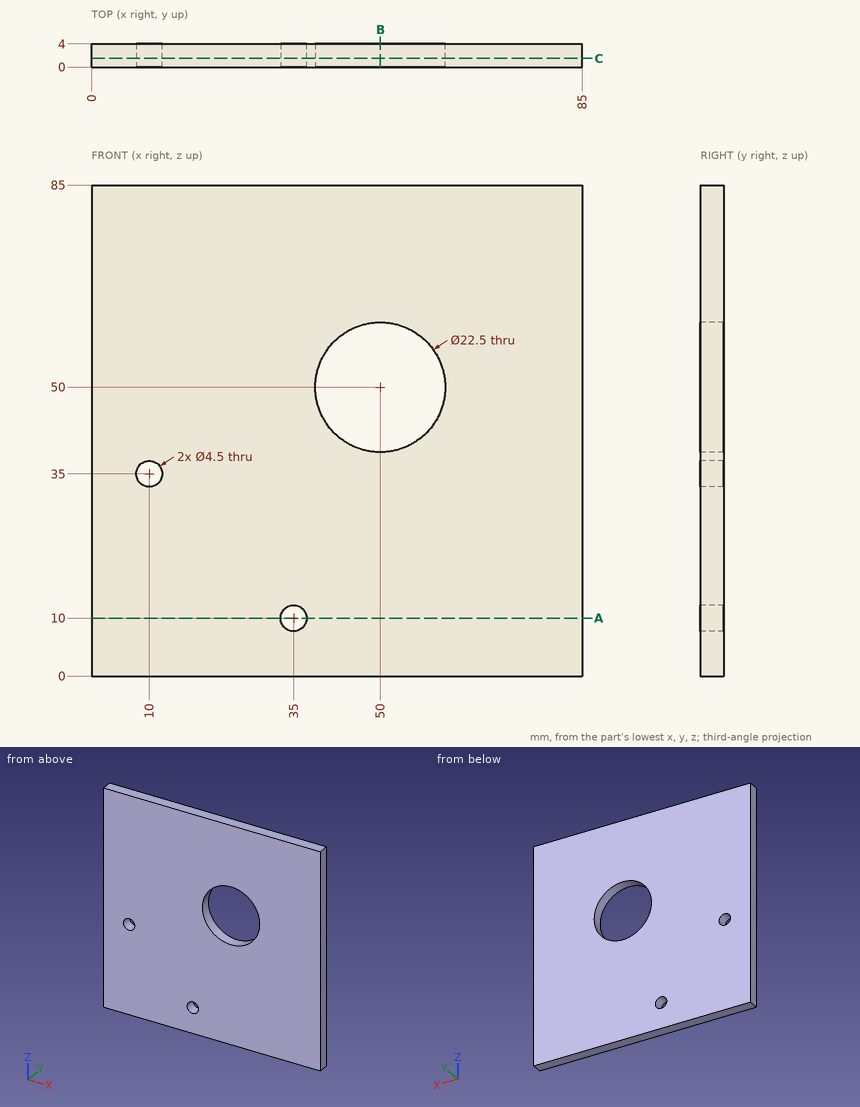
Here's the drawing with two shaded views (mm, measured from the low corner). I have some questions. Coordinates: 2 decimals unless noted, no trailing zeros. Loops run counter-clockwise (first coordinate to the right, second up) from the corner with the lowest first, then second, coordinate; pieces in that order, holes last. Notation, with made-up numbers: (41.25, 55) -> (46.25, 55) arc R18 ccw to (46.25, 62) -> close; hole circle Ø8 at (23.5, 24.5). An arc over 180 degrees is marked (long way). Put each result on its own line as item: value. Start each with the question number.
Q1. I want a section at A-A (z = 10). Write out the boundary of the cut face in (x, y).
Q2. I want a section at C-C (y = 1.5). Write out the boundary of the cut face in (x, z), plus the area to 3 significant figures.
Q3. If I drill on line 1 (Z direction, x = 50, y = 2.9); line 2 (Z direction, x = 10, y = 2.4), over which ranges is the centre line in solid material (lowest first)? Write a range as [from, to].
Q4. I want a section at B-B (x = 50). Write out the boundary of the cut face in (y, z), plus the area to 3 significant figures.
Taken from the geometry:
1. outline: (0, 0) -> (32.75, 0) -> (32.75, 4) -> (0, 4) -> close; (37.25, 0) -> (85, 0) -> (85, 4) -> (37.25, 4) -> close
2. outline: (0, 0) -> (85, 0) -> (85, 85) -> (0, 85) -> close; hole circle Ø4.5 at (10, 35); hole circle Ø4.5 at (35, 10); hole circle Ø22.5 at (50, 50)
2. area: 6,800 mm2
3. line 1: z = [0, 38.75], [61.25, 85]
3. line 2: z = [0, 32.75], [37.25, 85]
4. outline: (0, 0) -> (4, 0) -> (4, 38.75) -> (0, 38.75) -> close; (0, 61.25) -> (4, 61.25) -> (4, 85) -> (0, 85) -> close
4. area: 250 mm2
